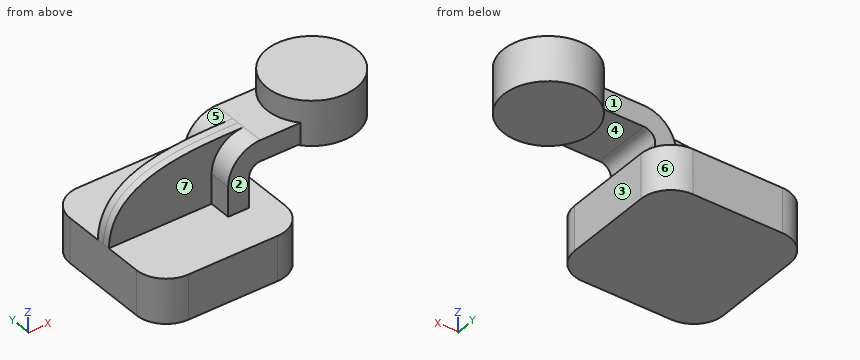
```python
from build123d import *

# Parameters (mm, degrees)
F1_DEPTH = 63.5
F2_DEPTH = 6.35
F0_W     = 38.1
F0_H     = 17.78
F3_DEPTH = 25.4
F5_R     = 25.4


with BuildPart() as f1:
    # F0 (on Front) → F1 (new body, symmetric)
    with BuildSketch(Plane.XZ):
        Polygon((63.5, -19.05), (63.5, 19.05), (41.950526, 19.05), (24.170526, 19.05), (-63.5, 19.05), (-63.5, -19.05), align=None)
    extrude(amount=F1_DEPTH, both=True)

    # F0 (on Front) → F2 (join, symmetric)
    with BuildSketch(Plane.XZ):
        with BuildLine():
            Line((-63.5, 19.05), (24.170526, 19.05))
            Line((24.170526, 19.05), (24.170526, 44.45))
            ThreePointArc((24.170526, 44.45), (32.219419, 63.881746), (51.651164, 71.930638))
            add(Edge.make_bspline(
                [(-63.5, 19.05), (-61.917547, 72.500213), (3.013055, 72.448058), (51.651164, 71.930638)],
                knots=[0, 0, 0, 0, 126.712874, 126.712874, 126.712874, 126.712874], degree=3))
        make_face()
    extrude(amount=F2_DEPTH, both=True)

    # F0 (on Front) → F3 (join, symmetric)
    with BuildSketch(Plane.XZ):
        with BuildLine():
            Line((24.170526, 19.05), (41.950526, 19.05))
            Line((41.950526, 19.05), (41.950526, 44.45))
            ThreePointArc((41.950526, 44.45), (44.791777, 51.309387), (51.651164, 54.150638))
            Line((51.651164, 54.150638), (76.2, 54.150638))
            Line((76.2, 54.150638), (76.2, 71.930638))
            Line((76.2, 71.930638), (51.651164, 71.930638))
            ThreePointArc((51.651164, 71.930638), (32.219419, 63.881746), (24.170526, 44.45))
            Line((24.170526, 44.45), (24.170526, 19.05))
        make_face()
        with Locations((95.25, 63.040638)):
            Rectangle(F0_W, F0_H)
    extrude(amount=F3_DEPTH, both=True)

    # F0 (on Front) → F4 (revolve)
    with BuildSketch(Plane.XZ):
        Polygon((114.3, 71.930638), (114.3, 54.150638), (114.3, 52.880638), (152.4, 52.880638), (152.4, 90.980638), (114.3, 90.980638), align=None)
    revolve(axis=Axis((114.3, 0, 71.930638), (0, 0, 1)))

    # F5
    f5_edges = [f1.edges().sort_by_distance(p)[0] for p in [
        (-63.5, -63.5, 0),
        (63.5, -63.5, 0),
        (-63.5, 63.5, 0),
        (63.5, 63.5, 0),
    ]]
    fillet(f5_edges, radius=F5_R)


solid = f1.part
```
The listing builds one solid part. Answer for the finished solid, in the listing's coordinates (mm). Face numbers are marked on the shaded views. A direction names the side the tool comes from. Coordinates: 2 decimals unless noted, no trailing zeros. Loops run counter-clockwise (first coordinate to the right, second up) from the corner with the lowest first, then second, coordinate; pieces in that order, holes last. Notation, with made-up numbers: M -22.5,48.25 L 23.5,48.25 A10 cw 23.5,67.25 Z; hole C 0,-40 d1. An arc over 180 degrees is marked long. Answer as CSV lines item,"result". Start each with the question number.
(1) The part is cut by section C-C (z = 3.5). Give the vertices of the cut face in (x, y).
(2) The part is cut by section B-B (x = 61). Give the vertices of the cut face in (y, z).
(3) The part is cut by section A-A (y = -35). Give the vertices of the cut face in (x, z), and give its area (3 significant figures).
(4) The part is cut by section D-D (y = -16.5). Give the vertices of the cut face in (x, z), and give its area (3 significant figures).
(5) The mould has two halves that part along X. Classify the marked faces 4, 5, 6 and 7: pulls with the +X half, pulls with the -X half, needs draft (parallel to the pull), parting line crosses it, or undercut.
(6) Find the intervals of material crossed by L1, parallel to Z at x = -27, y = 34.5; L2, parallel to X at y = 23, z = 31.5; L3, parallel to X at y = -15, z = 2.5, in increasing order. Write a range as [from, to].
(7) Given pin 1 (5 mm diameter, centred on x = 64, y = 11.5, fed in from +Z); pin 2 (10 mm diameter, centred on y = 47.5, z = 58.5, fed in from -X); pin 3 (1 mm diameter, centred on y = -13, z = 62, fed in from -X); pin 4 (21 mm diameter, centred on y = -20, z = 30.5, fed in from -X), each flat-ended and moving along its own axis, determine where each tip first touches the part or whether it passes through.
(8) For the marked faces 1, 2 and 3, determine the directions among +Z, -Z, +X, -X, +Y, -Y from which every point of the face is accessible in a straight line to the end or side of a thin tool.
Determined:
1,outline,"M -63.5,-38.1 A25.4 ccw -38.1,-63.5 L 38.1,-63.5 A25.4 ccw 63.5,-38.1 L 63.5,38.1 A25.4 ccw 38.1,63.5 L -38.1,63.5 A25.4 ccw -63.5,38.1 Z"
2,outline,"M -49.09,-19.05 L 49.09,-19.05 L 49.09,19.05 L -49.09,19.05 Z; M -25.4,54.15 L 25.4,54.15 L 25.4,71.93 L -25.4,71.93 Z"
3,outline,"M -63.5,-19.05 L 63.5,-19.05 L 63.5,19.05 L -63.5,19.05 Z; M 99.25,52.88 L 129.35,52.88 L 129.35,90.98 L 99.25,90.98 Z"
3,area,"5,990 mm2"
4,outline,"M -63.5,-19.05 L 63.5,-19.05 L 63.5,19.05 L 41.95,19.05 L 41.95,44.45 A9.7 cw 51.65,54.15 L 79.96,54.15 L 79.96,52.88 L 148.64,52.88 L 148.64,90.98 L 79.96,90.98 L 79.96,71.93 L 51.65,71.93 A27.48 ccw 24.17,44.45 L 24.17,19.05 L -63.5,19.05 Z"
4,area,"8,930 mm2"
5,face 4,"undercut"
5,face 5,"pulls with the -X half"
5,face 6,"pulls with the +X half"
5,face 7,"needs draft"
6,L1,"[-19.05, 19.05]"
6,L2,"[24.17, 41.95]"
6,L3,"[-63.5, 63.5]"
7,pin 1,"z = 71.93"
7,pin 2,"through"
7,pin 3,"x = 30.1"
7,pin 4,"x = 24.17"
8,face 1,"+Z, -X, +Y"
8,face 2,"+Z, -X, -Y"
8,face 3,"-Z, +X, +Y, -Y"
